from build123d import *

# Parameters (mm, degrees)
ESQUISSE1_R             = 5
BOSS_EXTRU_1_DEPTH      = 2
ESQUISSE2_R             = 1.5
ENL_V_MAT_EXTRU_2_DEPTH = 13
ESQUISSE3_R             = 3.5
ENL_V_MAT_EXTRU_4_DEPTH = 1
CONG_1_R                = 1


with BuildPart() as part:
    # Esquisse1 → Boss.-Extru.1 (new body)
    with BuildSketch(Plane.XY):
        Circle(ESQUISSE1_R)
    extrude(amount=BOSS_EXTRU_1_DEPTH)

    # Esquisse2 → Enlèv. mat.-Extru.2 (cut)
    with BuildSketch(Plane.XY):
        Circle(ESQUISSE2_R)
    extrude(amount=ENL_V_MAT_EXTRU_2_DEPTH, mode=Mode.SUBTRACT)

    # Esquisse3 → Enlèv. mat.-Extru.4 (cut)
    with BuildSketch(Plane.XY):
        Circle(ESQUISSE3_R)
    extrude(amount=ENL_V_MAT_EXTRU_4_DEPTH, mode=Mode.SUBTRACT)

    # Congé1
    cong_1_edges = [part.edges().sort_by_distance(p)[0] for p in [
        (-5, 0, 0),
    ]]
    fillet(cong_1_edges, radius=CONG_1_R)


solid = part.part
Model file for the job. Use its own axes, mm. A direction names the side the tool comes from. Give positions to 0.01 mm unless a question says otherwise; leave off trailing zeros. Loops run counter-clockwise (first coordinate to the right, second up) from the corner with the lowest first, then second, coordinate; pieces in that order, holes last.
1) Tool access for faces 4 (the cylindrical face through (3.233, -1.341, 0.493)), 5 (the cylindrical face through (-1.5, 0.07, 1.49)): list every direction of +Z, -Z, +X, -X, +Y, -Y with a clear straight run to the whole face (end or side of a thin tool).
2) Saw through at B-B (z = 1.7). Write the cut outline in (x, y).
3) Saw through at C-C (z = 0.35). Write the cut outline in (x, y), plus the area to 3 significant figures.
4) Wall check: line 1 (Y direction, x = 0, z = 1.55); line 2 (Z direction, x = 2.5, y = -2); line 3 (Y direction, x = 0, z = 0.6). Give the ranges that are in metal, low to high.
5) Pull direction X, two halves, no side cores. Call faces 1 (the cylindrical face through (-1.08, -4.88, 1.49)), 2 (the flat face through (0, -2, 1)), 3 (the flat face through (-1.2, 1.2, 2)): +X half, -X half, draft (parallel to the pull), parting line (faces both ways), or undercut.
6) Saw through at A-A (x = 0). Write the cut outline in (y, z).
7) Flat gauge pin, fed straight in: pin 1 Ø3.5 at (x, y) = (-0.5, -0.5) entering from -Z. Where does the tip first touch, or does it go through?
Answer block:
1. face 4: -Z
1. face 5: +Z, -Z
2. outline: circle Ø10 at (0, 0); hole circle Ø3 at (0, 0)
3. outline: circle Ø9.52 at (0, 0); hole circle Ø7 at (0, 0)
3. area: 32.7 mm2
4. line 1: y = -5 to -1.5, 1.5 to 5
4. line 2: z = 1 to 2
4. line 3: y = -4.92 to -3.5, 3.5 to 4.92
5. face 1: parting line
5. face 2: undercut
5. face 3: draft
6. outline: (-5, 1) arc R1 ccw to (-4, 0) - (-3.5, 0) - (-3.5, 1) - (-1.5, 1) - (-1.5, 2) - (-5, 2) - close; (1.5, 1) - (3.5, 1) - (3.5, 0) - (4, 0) arc R1 ccw to (5, 1) - (5, 2) - (1.5, 2) - close
7. pin 1: stops at z = 1
